Could you check a few things on this model? Use its own coordinates, in mm. Face numbers are marked on the shaded views. A direction names the side the tool comes from. Coordinates: 2 decimals unless noted, no trailing zeros. Order: outer loops, then holes, each group sorted by start corner. A loop starts at its lowest first (then second) coordinate and runs counter-clockwise, first axis right, second up. Notation, with made-up numbers: (13, -32.75) - (45, -32.75) arc R33 cw to (45, 6.25) - close; hole circle Ø3 at (77, 7.25). An arc over 180 degrees is marked (long way). One line per item, written item: value.
Autodesk Fusion 360 part; units mm, degrees
sketch "Sketch1" plane through (0, 0, 0) normal (0, 0, 1) x (1, 0, 0)
  line L0 (0, 0) -> (30, 0)
  line L1 (30, 0) -> (30, 35)
  line L2 (30, 35) -> (0, 35)
  line L3 (0, 35) -> (0, 0)
  dimension "d1" = 30
  dimension "d2" = 35
extrude "Extrude1" add sketch "Sketch1" along normal blind 30
sketch "Sketch2" plane through (0, 0, 0) normal (0, 0, -1) x (1, 0, 0)
  line L0 (0, 0) -> (0, -35)
  line L1 (0, -35) -> (30, -35)
  line L2 (30, -35) -> (30, 0)
  line L3 (30, 0) -> (0, 0)
  line L4 (30, 0) -> (0, 0)
  line L5 (0, 0) -> (0, -5)
  line L6 (0, -5) -> (30, -5)
  line L7 (30, -5) -> (30, 0)
  line L8 (30, -35) -> (0, -35)
  line L9 (0, -35) -> (0, -30)
  line L10 (0, -30) -> (30, -30)
  line L11 (30, -30) -> (30, -35)
extrude "Extrude2" cut sketch "Sketch2" against normal blind 4 contours L0 L2 L3 L4 L5 L6 L7 | L0 L1 L2 L8 L9 L10 L11
sketch "Sketch3" plane through (0, 5, 0) normal (0, -1, 0) x (1, 0, 0)
  line L0 (0, 0) -> (30, 0)
  line L1 (30, 0) -> (30, 4)
  line L2 (30, 4) -> (0, 4)
  line L3 (0, 4) -> (0, 0)
  line L4 (0, 4) -> (5, 0)
extrude "Extrude3" cut sketch "Sketch3" against normal blind 100 contours L0 L3 L4
sketch "Sketch4" plane through (0, 5, 0) normal (0, -1, 0) x (1, 0, 0)
  line L0 (0, 4) -> (5, 0)
  line L1 (5, 0) -> (30, 0)
  line L2 (30, 0) -> (30, 4)
  line L3 (30, 4) -> (0, 4)
  circle A0 centre (7, 2.5) radius 1
  dimension "d9" = 2
sketch "Sketch5" plane through (0, 0, 0) normal (0, 0, -1) x (1, 0, 0)
  line L0 (5, -5) -> (5, -30)
  line L1 (5, -30) -> (30, -30)
  line L2 (30, -30) -> (30, -5)
  line L3 (30, -5) -> (5, -5)
  line L4 (25, -26) -> (10, -26)
  line L5 (10, -26) -> (10, -9)
  line L6 (10, -9) -> (25, -9)
  line L7 (25, -9) -> (25, -26)
extrude "Extrude5" cut sketch "Sketch5" against normal blind 100 contours L4 L5 L6 L7
sketch "Sketch6" plane through (25, 0, 0) normal (-1, 0, 0) x (0, -1, 0)
  line L0 (-9, 30) -> (-26, 30)
  line L1 (-26, 30) -> (-26, 0)
  line L2 (-26, 0) -> (-9, 0)
  line L3 (-9, 0) -> (-9, 30)
  line L4 (-9, 0) -> (-26, 0)
  line L5 (-26, 0) -> (-26, 3)
  line L6 (-26, 3) -> (-9, 3)
  line L7 (-9, 3) -> (-9, 0)
  dimension "d14" = 17
  dimension "d15" = 3
extrude "Extrude6" add sketch "Sketch6" along normal blind 5 contours L1 L2 L3 L4 L5 L6 L7
sketch "Sketch7" plane through (0, 0, 0) normal (0, -1, 0) x (1, 0, 0)
  line L0 (0, 4) -> (30, 4)
  line L1 (30, 4) -> (30, 30)
  line L2 (30, 30) -> (0, 30)
  line L3 (0, 30) -> (0, 4)
  line L4 (0, 25) -> (6, 30)
extrude "Extrude7" cut sketch "Sketch7" against normal blind 100 contours L2 L3 L4
sketch "Sketch8" plane through (0, 0, 30) normal (0, 0, 1) x (-1, 0, 0)
  line L0 (-6, -35) -> (-6, 0)
  line L1 (-6, 0) -> (-30, 0)
  line L2 (-30, 0) -> (-30, -35)
  line L3 (-30, -35) -> (-6, -35)
  line L4 (-10, -9) -> (-10, -26)
  line L5 (-10, -26) -> (-25, -26)
  line L6 (-25, -26) -> (-25, -9)
  line L7 (-25, -9) -> (-10, -9)
  line L8 (-30, -30) -> (0, -30)
  line L9 (0, -30) -> (0, -5)
  line L10 (0, -5) -> (-30, -5)
  line L11 (-30, -5) -> (-30, -30)
extrude "Extrude8" cut sketch "Sketch8" against normal blind 5 contours L0 L2 L8 L10 L11 | L0 L8 L9 L10
sketch "Sketch9" plane through (0, 5, 0) normal (0, -1, 0) x (1, 0, 0)
  line L0 (0, 4) -> (5, 0)
  line L1 (5, 0) -> (30, 0)
  line L2 (30, 0) -> (30, 4)
  line L3 (30, 4) -> (0, 4)
  circle A0 centre (7, 2) radius 0.8
  dimension "d22" = 1.6
extrude "Extrude9" cut sketch "Sketch9" against normal blind 100 contours A0
sketch "Sketch10" plane through (0, 0, 0) normal (0, -1, 0) x (1, 0, 0)
  line L0 (6, 30) -> (0, 25)
  line L1 (0, 25) -> (0, 4)
  line L2 (0, 4) -> (30, 4)
  line L3 (30, 4) -> (30, 30)
  line L4 (30, 30) -> (6, 30)
  circle A0 centre (7, 28.5) radius 0.8
  dimension "d25" = 1.6
sketch "Sketch11" plane through (0, 0, 0) normal (0, -1, 0) x (1, 0, 0)
  line L0 (6, 30) -> (0, 25)
  line L1 (0, 25) -> (0, 4)
  line L2 (0, 4) -> (30, 4)
  line L3 (30, 4) -> (30, 30)
  line L4 (30, 30) -> (6, 30)
  circle A0 centre (7, 27.545) radius 0.8
  line L5 (7, 27.545) -> (7, 1)
  dimension "d28" = 1.6
  dimension "d29" = 7
  dimension "d30" = 2.455
extrude "Extrude11" cut sketch "Sketch11" against normal blind 100 contours A0
sketch "Sketch12" plane through (10, 0, 0) normal (1, 0, 0) x (0, 1, 0)
  line L0 (26, 25) -> (9, 25)
  line L1 (9, 25) -> (9, 0)
  line L2 (9, 0) -> (26, 0)
  line L3 (26, 0) -> (26, 25)
  line L4 (26, 0) -> (9, 0)
  line L5 (9, 0) -> (9, 3)
  line L6 (9, 3) -> (26, 3)
  line L7 (26, 3) -> (26, 0)
  dimension "d33" = 17
  dimension "d34" = 3
extrude "Extrude12" add sketch "Sketch12" along normal blind 2 contours L1 L2 L3 L4 L5 L6 L7
extrude "Extrude13" cut 1 faces at (20, 20.3333, 1) along direction (1, 0, 0) blind 2.5
extrude "Extrude14" cut 1 faces at (24.1667, 20.3333, 3) along direction (0, 0, -1) blind 1
extrude "Extrude15" cut 1 faces at (10.6667, 14.6667, 3) along direction (0, 0, -1) blind 1
extrude "Extrude16" cut 2 faces at (10.6667, 14.6667, 2) (24.1667, 20.3333, 2) along direction (0, 0, -1) blind 0.5
extrude "Extrude17" add 1 faces at (12, 14.6667, 0.5) along direction (1, 0, 0) blind 0.5
extrude "Extrude18" cut 1 faces at (10, 20.3333, 9.8333) along direction (-1, 0, 0) blind 2
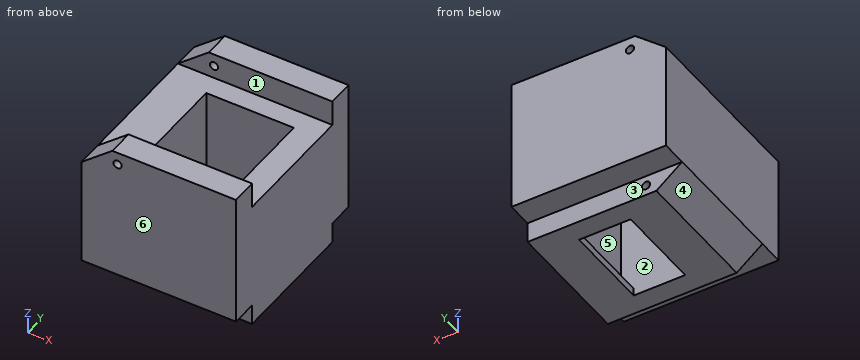
Item 1: I want a section at C-C on x = 7. Please give me the cut outline in (y, z) (3 decimals), then the cut area to 3 significant figures.
Conclusion:
outline: (0, 4) - (5, 4) - (5, 2.8) - (30, 2.8) - (30, 4) - (35, 4) - (35, 26.745) - (30, 26.745) - (30, 25) - (5, 25) - (5, 26.745) - (0, 26.745) - close; (0, 28.345) - (5, 28.345) - (5, 30) - (0, 30) - close; (5, 0) - (30, 0) - (30, 1.2) - (5, 1.2) - close; (30, 28.345) - (35, 28.345) - (35, 30) - (30, 30) - close
area: 829 mm²
Item 2: I'm going to push flat-ended pins straight in: pin 1 Ø1.8 at (x, z) = (7, 2) entering from +Y; pin 2 Ø2 at (x, y) = (9.5, 17) entering from +Z; pin 3 Ø2.5 at (x, y) = (12.5, 33) entering from -Z. Where does each tip first touch, or does it pass through?
Conclusion:
pin 1: y = 30
pin 2: z = 1.5
pin 3: z = 4
Item 3: I want a section at A-A on z = 2. Please give me the cut outline in (x, y), then the cut area to 4 significant figures.
Conclusion:
outline: (2.5, 5) - (6.2, 5) - (6.2, 30) - (2.5, 30) - close; (7.8, 5) - (30, 5) - (30, 30) - (7.8, 30) - close; hole (8, 9) - (25, 9) - (25, 26) - (8, 26) - close
area: 358.5 mm²
Item 4: For the marked faces 1, 2 and 3, which set-ups out of +Z, -Z, +X, -X, +Y, -Y let a thin tool reach every point of the face, with its end or its side?
Conclusion:
face 1: +Z, +X, -X
face 2: +Z
face 3: -Z, +X, -X, +Y
Item 5: Thinking about a two-plate mould opening in Y: for the marked faces 4, 5 and 6, which applies, pulls with the +Y half, pulls with the -Y half, needs draft (parallel to the pull), parting line crosses it, or undercut?
Conclusion:
face 4: needs draft
face 5: undercut
face 6: pulls with the -Y half
Item 6: If I drill on probe 1 along Z at (x, y) = (7, 3.3) (3 decimals); probe 2 along Y at (x, z) = (23.25, 16); probe 3 along Y at (x, z) = (24.75, 26), over which ranges is the centre line in solid material (lowest first)?
Conclusion:
probe 1: 4 to 26.745, 28.345 to 30
probe 2: 0 to 9, 26 to 35
probe 3: 0 to 5, 30 to 35
Item 7: I want a section at B-B on y = 14. Please give me the cut outline in (x, z), then the cut area to 3 significant figures.
Conclusion:
outline: (0, 4) - (5, 0) - (12.5, 0) - (12.5, 1.5) - (8, 1.5) - (8, 25) - (0, 25) - close; (22.5, 0) - (30, 0) - (30, 25) - (25, 25) - (25, 1.5) - (22.5, 1.5) - close; hole circle Ø1.6 at (7, 2)
area: 323 mm²
Item 8: I want a section at D-D on z = 22.5. Please give me the cut outline in (x, y).
Conclusion:
outline: (0, 0) - (30, 0) - (30, 35) - (0, 35) - close; hole (8, 9) - (25, 9) - (25, 26) - (8, 26) - close
